Can you work these out from the model? Positions are in its coordinate system, mm. A direction names the side the tool comes from. Coordinates: 2 decimals unless noted, no trailing zeros. Order: outer loops, then holes, each group sorted by start corner. A loop starts at its lowest first (then second) coordinate and runs counter-clockwise, first axis right, second up.
```python
from build123d import *

# Parameters (mm, degrees)
F0_R     = 40.47
F0_R_2   = 38.145
F1_DEPTH = 5
F2_R     = 40.47
F3_DEPTH = 5
F4_R     = 5
F5_R     = 1


with BuildPart() as f1:
    # F0 (on Top) → F1 (new body)
    with BuildSketch(Plane.XY):
        Circle(F0_R)
        Circle(F0_R_2, mode=Mode.SUBTRACT)
    extrude(amount=F1_DEPTH)

    # F2 (on face) → F3 (join)
    with BuildSketch(Plane.XY.offset(5)):
        Circle(F2_R)
    extrude(amount=F3_DEPTH)

    # F4
    f4_edges = [f1.edges().sort_by_distance(p)[0] for p in [
        (-40.47, 0, 10),
    ]]
    fillet(f4_edges, radius=F4_R)

    # F5
    f5_edges = [f1.edges().sort_by_distance(p)[0] for p in [
        (-40.47, 0, 0),
    ]]
    fillet(f5_edges, radius=F5_R)


solid = f1.part
```
1. Imagine slicing it at A-A on x = 0. Please give me the cut outline in (y, z) (3 decimals).
Completed:
outline: (-40.47, 1) arc R1 ccw to (-39.47, 0) - (-38.145, 0) - (-38.145, 5) - (38.145, 5) - (38.145, 0) - (39.47, 0) arc R1 ccw to (40.47, 1) - (40.47, 5) arc R5 ccw to (35.47, 10) - (-35.47, 10) arc R5 ccw to (-40.47, 5) - close
2. I'm going to push flat-ended pins straight in: pin 1 (5 mm diameter, centred on x = 1, z = 3.5, fed in from -Y); pin 2 (6 mm diameter, centred on x = 12, z = 4, fed in from +Y); pin 3 (4 mm diameter, centred on x = 15.5, y = 18.5, fed in from -Z). Where does each tip first touch, or does it pass through?
Completed:
pin 1: stops at y = -40.47
pin 2: stops at y = 39.46
pin 3: stops at z = 5
3. Imagine slicing it at C-C on z = 8. Please give me the cut outline in (x, y), then the cut area to 3 significant figures.
Completed:
outline: circle Ø78.94 at (0, 0)
area: 4,890 mm2
4. Thinking about a two-plate mould opening in X: for faces 3 (the cylindrical face through (-30.27, -23.21, 2.46)), 4 (the flat face through (0, 0, 10)), 5 (the cylindrical face through (18.674, -35.904, 2.972)), which applies, pulls with the +X half, pulls with the -X half, needs draft (parallel to the pull), parting line crosses it, or undercut?
Completed:
face 3: undercut
face 4: needs draft
face 5: parting line crosses it
5. Please list where these lines run through material, in increasing order: probe 1 along Y at (x, z) = (0, 1) (3 decimals); probe 2 along Z at (x, y) = (9, 23); probe 3 along X at (y, z) = (16.5, 1.5).
Completed:
probe 1: y = -40.47 to -38.145, 38.145 to 40.47
probe 2: z = 5 to 10
probe 3: x = -36.95 to -34.39, 34.39 to 36.95
6. On a 3-axis mill with a long thin cutter (end or side, diameter ignored), from which of +Z, -Z, +X, -X, +Y, -Y can I reach the whole of each face in a straight line? I mean faces 1 (the flat face through (-20.7, 32.3, 0)), 2 (the flat face through (-1, 1, 5)). Say none if no direction works.
Completed:
face 1: -Z, +X, -X, +Y, -Y
face 2: -Z
7. Imagine slicing it at D-D on z = 3.5. Please give me the cut outline in (x, y) (3 decimals).
Completed:
outline: circle Ø80.94 at (0, 0); hole circle Ø76.29 at (0, 0)
